```python
from build123d import *

# Parameters (mm, degrees)
F1_DEPTH    = 10
F2_T1_DEPTH = 25
F3_SIZE     = 0.5


# Not quite as in the source:
# - a fillet or chamfer that OpenCascade refuses, or shapes differently, is made with other operations: its cross-section is extruded or revolved along the edge and cut away or added


with BuildPart() as f1:
    # F0 (on Top) → F1 (new body)
    with BuildSketch(Plane.XY):
        Polygon((-15, 4), (-15, 0), (-2.5, 0), (-2.5, -15), (2.5, -15), (2.5, 0), (15, 0), (15, 4), align=None)
    extrude(amount=F1_DEPTH)

    # F2: fillet of radius 3 on 4 edges, made by hand

    # F2_s2 → F2_t1 (cut)
    with BuildSketch(Plane.XY.offset(-7.5)):
        with BuildLine():
            ThreePointArc((-2.5, -12), (-1.6213203436, -14.1213203436), (0.5, -15))
            Line((0.5, -15), (-2.5, -15))
            Line((-2.5, -15), (-2.5, -12))
        make_face()
        with BuildLine():
            ThreePointArc((-0.5, -15), (1.6213203436, -14.1213203436), (2.5, -12))
            Line((2.5, -12), (2.5, -15))
            Line((2.5, -15), (-0.5, -15))
        make_face()
        with BuildLine():
            ThreePointArc((-15, 3), (-14.1213203436, 0.8786796564), (-12, 0))
            Line((-12, 0), (-15, 0))
            Line((-15, 0), (-15, 3))
        make_face()
        with BuildLine():
            ThreePointArc((12, 0), (14.1213203436, 0.8786796564), (15, 3))
            Line((15, 3), (15, 0))
            Line((15, 0), (12, 0))
        make_face()
    extrude(amount=F2_T1_DEPTH, mode=Mode.SUBTRACT)

    # F3
    f3_edges = [f1.edges().sort_by_distance(p)[0] for p in [
        (0, 4, 10),
        (15, 3.5, 10),
        (14.12132, 0.87868, 10),
        (7.25, 0, 10),
        (2.5, -6, 10),
        (1.791288, -13.936492, 10),
        (-1.791288, -13.936492, 10),
        (-2.5, -6, 10),
        (-7.25, 0, 10),
        (-14.12132, 0.87868, 10),
        (-15, 3.5, 10),
        (0, 4, 0),
        (15, 3.5, 0),
        (14.12132, 0.87868, 0),
        (7.25, 0, 0),
        (2.5, -6, 0),
        (1.791288, -13.936492, 0),
        (-1.791288, -13.936492, 0),
        (-2.5, -6, 0),
        (-7.25, 0, 0),
        (-14.12132, 0.87868, 0),
        (-15, 3.5, 0),
    ]]
    chamfer(f3_edges, length=F3_SIZE)


solid = f1.part
```
Geometry check sheet. Reference: the model listing, model coordinates, mm. A direction names the side the tool comes from. Round coordinates to 2 decimals unless told otherwise and drop trailing zeros. Order: outer loops, then holes, each group sorted by start corner. A loop starts at its lowest first (then second) coordinate and runs counter-clockwise, first axis right, second up. Notation, with made-up numbers: (42.5, 29.5) - (95.5, 29.5) arc R19 ccw to (95.5, 39.5) - close; hole circle Ø11 at (72.25, 31). An arc over 180 degrees is marked (long way). Use a Markdown table: item, result. Add a question column.
1) Set-up check for faces 1 (the flat face through (-7, 0, 5)), 2 (the conical face through (1.501, -13.725, 9.858)), 3 (the flat face through (7, 0, 5)): record each of +Z, -Z, +X, -X, +Y, -Y from which the full face is reachable in a straight line by a thin tool's end or side.
2) Section check B-B (x = 11.5). Record the cut outline in (y, z), then the cut area to 3 significant figures.
3) Section check A-A (z = 2.25). Record the cut outline in (x, y), then the cut area to 3 significant figures.
4) Gauge pin test, flat ends, axial feed: P1, Ø2, axis at y = -3, z = 7, coming from the -X side; P2, Ø3, axis at x = 5, y = -8.5, coming from the -Z side; P3, Ø4.5, axis at x = 5.5, z = 5, coming from the -Y side. Record the tip position at first contact, or that the pin passes through.
5) Thickness scan on line 1 along Y through (x, z) = (-6.5, 9.5); line 2 along X through (y, z) = (-8, 2); line 3 along Y through (x, z) = (-2.25, 4.5). Record the ranges inside material, lowest first.
6) Section check C-C (y = -2.75). Record the cut outline in (x, z), then the cut area to 3 significant figures.
Established:
| question | item | result |
|---|---|---|
| 1 | face 1 | +Z, -Z, -X, -Y |
| 1 | face 2 | +Z, +X, -Y |
| 1 | face 3 | +Z, -Z, +X, -Y |
| 2 | outline | (0, 0.5) - (0.5, 0) - (3.5, 0) - (4, 0.5) - (4, 9.5) - (3.5, 10) - (0.5, 10) - (0, 9.5) - close |
| 2 | area | 39.5 mm2 |
| 3 | outline | (-15, 3) arc R3 ccw to (-12, 0) - (-2.5, 0) - (-2.5, -12) arc R3 ccw to (0, -14.96) arc R3 ccw to (2.5, -12) - (2.5, 0) - (12, 0) arc R3 ccw to (15, 3) - (15, 4) - (-15, 4) - close |
| 3 | area | 187 mm2 |
| 4 | P1 | x = -2.5 |
| 4 | P2 | through |
| 4 | P3 | y = 0 |
| 5 | line 1 | 0 to 4 |
| 5 | line 2 | -2.5 to 2.5 |
| 5 | line 3 | -13.2 to 4 |
| 6 | outline | (-2.5, 0.5) - (-2, 0) - (2, 0) - (2.5, 0.5) - (2.5, 9.5) - (2, 10) - (-2, 10) - (-2.5, 9.5) - close |
| 6 | area | 49.5 mm2 |
